Verification items for the finished model (mm, model axes). Face numbers are marked on the shaded views. Coordinates: 2 decimals unless noted, no trailing zeros. Order: outer loops, then holes, each group sorted by start corner. A loop starts at its lowest first (then second) coordinate and runs counter-clockwise, first axis right, second up. Notation, with made-up numbers: (-24.5, 75.5) -> (2.5, 75.5) arc R23 ccw to (2.5, 113.5) -> close; hole circle Ø11 at (23.5, 41). An arc over 180 degrees is marked (long way). Write item = value, one per line. Start each with the question number.
1. Thickness scan on line 1 along Y through (x, z) = (24.5, 1.75); line 2 along X through (y, z) = (26.5, 1); line 3 along Y through (x, z) = (28.5, 2.75). Record the ranges inside material, lowest first. Write a range as from..to.
2. Cross-section at C-C on z = 5.75. Record the cut outline in (x, y), plus the area to 3 significant figures.
3. Cross-section at A-A on x = 36. Record the cut outline in (y, z).
4. Cross-section at D-D on y = 98. Record the cut outline in (x, z), plus the area to 3 significant figures.
5. Go/stop test with flat-tipped pins: P1, Ø4, axis at y = 19, z = 1.5, coming from the +X side; P2, Ø1.6, axis at x = 69.5, z = 1, coming from the +Y side; P3, Ø4.5, axis at x = 67.5, y = 8, coming from the +Z side. Record where each tip stops, or that it passes through.
6. Release check for a two-part mould opening along Y. For the marked faces 1 and 2 record: +Y half, -Y half, draft (parallel to the pull), parting line (faces both ways), or undercut.
7. Cross-section at B-B on y = 60.5. Record the cut outline in (x, z).
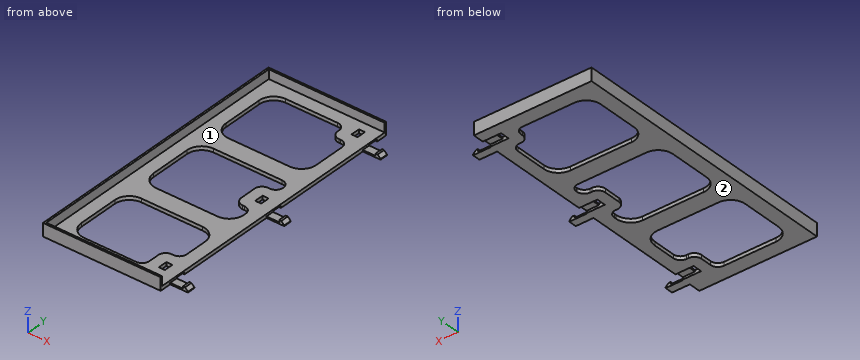
from build123d import *

# Parameters (mm, degrees)
F0_W      = 64.5
F0_H      = 151
F1_DEPTH  = 2
F3_DEPTH  = 5
F4_W      = 5
F4_H      = 1.2
F5_DEPTH  = 10
F6_W      = 4.3
F6_H      = 0.8
F7_DEPTH  = 9.75
F8_W      = 2.75
F8_H      = 4.3
F9_DEPTH  = 1.2
F10_W     = 2.75
F10_H     = 4.3
F11_DEPTH = 1.2
F12_W     = 2.75
F12_H     = 4.3
F13_DEPTH = 1.2
F14_W     = 3.3
F14_H     = 5
F15_DEPTH = 5.801
F16_W     = 3.3
F16_H     = 5
F17_DEPTH = 5.801
F18_W     = 3.3
F18_H     = 5
F19_DEPTH = 5.801
F20_SIZE  = 1.6
F22_DEPTH = 2.001
F23_R     = 4
F24_R     = 8


with BuildPart() as f1:
    # F0 (on Top) → F1 (new body)
    with BuildSketch(Plane.XY):
        with Locations((32.25, 75.5)):
            Rectangle(F0_W, F0_H)
    extrude(amount=F1_DEPTH)

    # F2 (on face) → F3 (join)
    with BuildSketch(Plane.XY.offset(2)):
        Polygon((64.5, 150), (64.5, 151), (0, 151), (0, 0), (64.5, 0), (64.5, 1), (1, 1), (1, 150), align=None)
    extrude(amount=F3_DEPTH)

    # F4 (on face) → F5 (cut)
    with BuildSketch(Plane.YZ.offset(64.5)):
        with Locations((142.5, 0.6)):
            Rectangle(F4_W, F4_H)
        with Locations((78, 0.6)):
            Rectangle(F4_W, F4_H)
        with Locations((13.5, 0.6)):
            Rectangle(F4_W, F4_H)
    extrude(amount=-F5_DEPTH, mode=Mode.SUBTRACT)

    # F6 (on face) → F7 (join)
    with BuildSketch(Plane.YZ.offset(64.5)):
        with Locations((8.5, 0.4)):
            Rectangle(F6_W, F6_H)
        with Locations((73, 0.4)):
            Rectangle(F6_W, F6_H)
        with Locations((137.5, 0.4)):
            Rectangle(F6_W, F6_H)
    extrude(amount=F7_DEPTH)

    # F8 (on face) → F9 (join)
    with BuildSketch(Plane.XY.offset(0.8)):
        with Locations((72.875, 8.5)):
            Rectangle(F8_W, F8_H)
    extrude(amount=F9_DEPTH)

    # F10 (on face) → F11 (join)
    with BuildSketch(Plane.XY.offset(0.8)):
        with Locations((72.875, 73)):
            Rectangle(F10_W, F10_H)
    extrude(amount=F11_DEPTH)

    # F12 (on face) → F13 (join)
    with BuildSketch(Plane.XY.offset(0.8)):
        with Locations((72.875, 137.5)):
            Rectangle(F12_W, F12_H)
    extrude(amount=F13_DEPTH)

    # F14 (on face) → F15 (cut, through all)
    with BuildSketch(Plane(origin=(0, 0, 1.2), x_dir=(1, 0, 0), z_dir=(0, 0, -1))):
        with Locations((56.15, -13.5)):
            Rectangle(F14_W, F14_H)
    extrude(amount=-F15_DEPTH, mode=Mode.SUBTRACT)

    # F16 (on face) → F17 (cut, through all)
    with BuildSketch(Plane(origin=(0, 0, 1.2), x_dir=(1, 0, 0), z_dir=(0, 0, -1))):
        with Locations((56.15, -78)):
            Rectangle(F16_W, F16_H)
    extrude(amount=-F17_DEPTH, mode=Mode.SUBTRACT)

    # F18 (on face) → F19 (cut, through all)
    with BuildSketch(Plane(origin=(0, 0, 1.2), x_dir=(1, 0, 0), z_dir=(0, 0, -1))):
        with Locations((56.15, -142.5)):
            Rectangle(F18_W, F18_H)
    extrude(amount=-F19_DEPTH, mode=Mode.SUBTRACT)

    # F20
    f20_edges = [f1.edges().sort_by_distance(p)[0] for p in [
        (74.25, 8.5, 2),
        (74.25, 73, 2),
        (74.25, 137.5, 2),
    ]]
    chamfer(f20_edges, length=F20_SIZE)

    # F21 (on face) → F22 (cut, through all)
    with BuildSketch(Plane.XY.offset(2)):
        Polygon((8, 143), (8, 104.7), (57.5, 104.7), (57.5, 134), (48.5, 134), (48.5, 143), align=None)
        Polygon((8, 56.3), (57.5, 56.3), (57.5, 69.5), (48.5, 69.5), (48.5, 86.5), (57.5, 86.5), (57.5, 94.7), (8, 94.7), align=None)
        Polygon((8, 46.3), (8, 8), (48.5, 8), (48.5, 22), (57.5, 22), (57.5, 46.3), align=None)
    extrude(amount=-F22_DEPTH, mode=Mode.SUBTRACT)

    # F23
    f23_edges = [f1.edges().sort_by_distance(p)[0] for p in [
        (48.5, 134, 1),
        (48.5, 143, 1),
        (57.5, 134, 1),
        (57.5, 94.7, 1),
        (48.5, 86.5, 1),
        (48.5, 69.5, 1),
        (57.5, 69.5, 1),
        (48.5, 22, 1),
        (57.5, 86.5, 1),
        (57.5, 22, 1),
        (48.5, 8, 1),
    ]]
    fillet(f23_edges, radius=F23_R)

    # F24
    f24_edges = [f1.edges().sort_by_distance(p)[0] for p in [
        (8, 8, 1),
        (8, 56.3, 1),
        (8, 104.7, 1),
        (8, 46.3, 1),
        (8, 94.7, 1),
        (8, 143, 1),
        (57.5, 104.7, 1),
        (57.5, 56.3, 1),
        (57.5, 46.3, 1),
    ]]
    fillet(f24_edges, radius=F24_R)


solid = f1.part
Worked out:
q1.line_1 = 0..8, 46.3..56.3, 94.7..104.7, 143..151
q1.line_2 = 0..8, 57.5..64.5
q1.line_3 = 0..1, 150..151
q2.outline = (0, 0) -> (64.5, 0) -> (64.5, 1) -> (1, 1) -> (1, 150) -> (64.5, 150) -> (64.5, 151) -> (0, 151) -> close
q2.area = 278 mm²
q3.outline = (0, 0) -> (8, 0) -> (8, 2) -> (1, 2) -> (1, 7) -> (0, 7) -> close; (46.3, 0) -> (56.3, 0) -> (56.3, 2) -> (46.3, 2) -> close; (94.7, 0) -> (104.7, 0) -> (104.7, 2) -> (94.7, 2) -> close; (143, 0) -> (151, 0) -> (151, 7) -> (150, 7) -> (150, 2) -> (143, 2) -> close
q4.outline = (0, 0) -> (64.5, 0) -> (64.5, 2) -> (1, 2) -> (1, 7) -> (0, 7) -> close
q4.area = 134 mm²
q5.P1 = 64.5
q5.P2 = 139.65
q5.P3 = 0.8
q6.face_1 = undercut
q6.face_2 = draft
q7.outline = (0, 0) -> (8.96, 0) -> (8.96, 2) -> (1, 2) -> (1, 7) -> (0, 7) -> close; (56.54, 0) -> (64.5, 0) -> (64.5, 2) -> (56.54, 2) -> close
